Part model, mm, in its own coordinate system. Coordinates: 2 decimals unless noted, no trailing zeros. Loops run counter-clockwise (first coordinate to the right, second up) from the corner with the lowest first, then second, coordinate; pieces in that order, holes last. Notation, with made-up numbers: M 26,37.25 L 38,37.25 A9 ccw 38,46.25 Z; hole C 84.25,-37.5 d6. An arc over 180 degrees is marked long. Answer as a JSON object with one key per item and string values. Group by question number.
1. Saw through at B-B on y = 1. Write the cut outline in (x, z) (3 decimals), then the cut area to 3 significant figures.
2. Drill centre lines: L1, parallel to Y at x = -9.5, z = 1.8 (3 decimals); L2, parallel to Z at x = 0, y = 5.5; L3, parallel to Z at x = 1.5, y = -6. Where is each one in solid material? Low to high.
3. Saw through at D-D on x = -11. Write the cut outline in (y, z), then the cut area to 3 significant figures.
4. Mould opens along Y. For faces 1 (the face through (-18, 1, -36)), 2 (the face through (-10, 1, 3)), 3 (the face through (0, -7.5, -4)) say: released by +Y, released by -Y, zero draft, split by the parting line, or undercut.
5. Drop flat-ended pins along their axis: pin 1 Ø3 at (x, y) = (-9.5, 0) entering from -Z; pin 2 Ø5 at (y, z) = (-2.5, -18) entering from -X; pin 3 Ø3 at (y, z) = (5, -20) entering from +X. Give the stop position or say it passes through.
6. Saw through at C-C on z = -45. Write the cut outline in (x, y) (3 decimals).
7. Saw through at A-A on x = 0. Write the cut outline in (y, z).
from build123d import *

# Parameters (mm, degrees)
F1_R          = 18
F1_R_2        = 3.25
F2_DEPTH      = 7.5
F2_DEPTH_BACK = 9.5
F3_R          = 8.5
F3_R_2        = 5.225
F4_DEPTH      = 60
F5_DEPTH      = 60.0010001
F5_DEPTH_BACK = 3
F6_DEPTH      = 7.5010001009
F6_DEPTH_BACK = 9.5010001
F8_DEPTH      = 50


# Not quite as in the source:
# - a feature of the source that left no trace in its solid (it failed there, or was rolled back) is left out


with BuildPart() as f2:
    # F1 (on Front) → F2 (new body, two sides)
    with BuildSketch(Plane.XZ) as f2_sk:
        Circle(F1_R)
        Circle(F1_R_2, mode=Mode.SUBTRACT)
    extrude(amount=F2_DEPTH)
    extrude(f2_sk.sketch, amount=-F2_DEPTH_BACK)

    # F3 (on Top) → F4 (join)
    with BuildSketch(Plane.XY):
        with Locations((-9.5, 1)):
            Circle(F3_R)
        with Locations((-9.5, 1)):
            Circle(F3_R_2, mode=Mode.SUBTRACT)
        with Locations((-9.5, 1)):
            Circle(F3_R_2)
    extrude(amount=-F4_DEPTH)

    # F3 (on Top) → F5 (cut, two sides)
    with BuildSketch(Plane.XY) as f5_sk:
        with Locations((-9.5, 1)):
            Circle(F3_R_2)
    extrude(amount=-F5_DEPTH, mode=Mode.SUBTRACT)
    extrude(f5_sk.sketch, amount=F5_DEPTH_BACK, mode=Mode.SUBTRACT)

    # F1 (on Front) → F6 (cut, two sides)
    with BuildSketch(Plane.XZ) as f6_sk:
        Circle(F1_R_2)
    extrude(amount=F6_DEPTH, mode=Mode.SUBTRACT)
    extrude(f6_sk.sketch, amount=-F6_DEPTH_BACK, mode=Mode.SUBTRACT)

    # F1 (on Front) → F8 (cut, symmetric)
    with BuildSketch(Plane.XZ):
        Circle(F1_R_2)
    extrude(amount=F8_DEPTH, both=True, mode=Mode.SUBTRACT)


solid = f2.part
Outcome:
{
 "1": {"outline": "M -18,-60 L -14.725,-60 L -14.725,3 L -4.275,3 L -4.275,-60 L -1,-60 L -1,-17.972 A18 ccw long -18,0 Z; hole C 0,0 d6.5", "area": "1,110 mm²"},
 "2": {"L1": "y = -7.5 to -4.225, 6.225 to 9.5", "L2": "z = -18 to -3.25, 3.25 to 18", "L3": "z = -17.94 to -2.88, 2.88 to 17.94"},
 "3": {"outline": "M -7.5,-14.25 L -7.37,-14.25 L -7.37,-60 L -4.01,-60 L -4.01,3 L 6.01,3 L 6.01,-60 L 9.37,-60 L 9.37,-14.25 L 9.5,-14.25 L 9.5,14.25 L -7.5,14.25 Z", "area": "619 mm²"},
 "4": {"face 1": "split by the parting line", "face 2": "undercut", "face 3": "released by -Y"},
 "5": {"pin 1": "stops at z = 3", "pin 2": "stops at x = -17.94", "pin 3": "stops at x = -1.38"},
 "6": {"outline": "C -9.5,1 d17; hole C -9.5,1 d10.45"},
 "7": {"outline": "M -7.5,-18 L 9.5,-18 L 9.5,-3.25 L -7.5,-3.25 Z; M -7.5,3.25 L 9.5,3.25 L 9.5,18 L -7.5,18 Z"}
}
